Read the model definition and answer for the solid it produces. Units are mm, in the model's axes. Coordinates: 2 decimals unless noted, no trailing zeros. Write each loop counter-clockwise with the first axis right and the second up, starting at its lowest first coordinate (ties: lowest second). Pieces come first, ordered by that corner, then holes. Notation, with made-up numbers: (62.25, 30.25) -> (96.25, 30.25) arc R30 ccw to (96.25, 60.25) -> close; hole circle Ø1 at (42, 54). An arc over 180 degrees is marked (long way). Use CSV: the item, a comma, the result in double quotes.
from build123d import *

# Parameters (mm, degrees)
F0_W     = 13
F0_H     = 13
F1_DEPTH = 30
F2_SIZE  = 12.99999
F3_R     = 6.49999
F4_R     = 3
F5_DEPTH = 25
F6_SIZE  = 0.4


# Not quite as in the source:
# - a fillet or chamfer is up to 0.001 mm smaller than in the source, because OpenCascade refuses the exact size


with BuildPart() as f1:
    # F0 (on Top) → F1 (new body)
    with BuildSketch(Plane.XY):
        Rectangle(F0_W, F0_H)
    extrude(amount=F1_DEPTH)

    # F2 (size 13 in the source; OpenCascade refuses exactly that, so slightly less here)
    f2_edges = [f1.edges().sort_by_distance(p)[0] for p in [
        (0, -6.5, 0),
    ]]
    chamfer(f2_edges, length=F2_SIZE)

    # F3 (radius 6.5 in the source; OpenCascade refuses exactly that, so slightly less here)
    f3_edges = [f1.edges().sort_by_distance(p)[0] for p in [
        (6.5, 0, 30),
        (-6.5, 0, 30),
    ]]
    fillet(f3_edges, radius=F3_R)

    # F4 (on face) → F5 (cut)
    with BuildSketch(Plane(origin=(0, 6.5, 0), x_dir=(-1, 0, 0), z_dir=(0, 1, 0))):
        with Locations((0, 23.5)):
            Circle(F4_R)
    extrude(amount=-F5_DEPTH, mode=Mode.SUBTRACT)

    # F6
    f6_edges = [f1.edges().sort_by_distance(p)[0] for p in [
        (4.596197, 6.5, 28.096197),
        (4.596197, -6.5, 28.096197),
        (3, 6.5, 23.5),
        (3, -6.5, 23.5),
    ]]
    chamfer(f6_edges, length=F6_SIZE)


solid = f1.part
1. This flat-tipped pin is pushed along its axis until it touches: pin 1 Ø1.5 at (x, z) = (1, 9) entering from -Y. Where does it stop, or does it pass through?
Solutions:
pin 1,"stops at y = -3.25"
2. A cutting plane is placed at C-C (z = 2). Give the vertices of the cut face in (x, y), and give its area (3 significant figures).
Solutions:
outline,"(-6.5, 4.5) -> (6.5, 4.5) -> (6.5, 6.1) -> (6.1, 6.5) -> (-6.1, 6.5) -> (-6.5, 6.1) -> close"
area,"25.8 mm^2"
3. Find the intervals of material crossed by line 1 along Z through (x, y) = (0, 3.5); line 2 along Z through (x, y) = (-2.25, -4); line 3 along Y through (x, z) = (1.5, 6.5), in increasing order.
Solutions:
line 1,"z = 3 to 20.5, 26.5 to 30"
line 2,"z = 10.5 to 21.52, 25.48 to 29.6"
line 3,"y = 0 to 6.5"
4. A cutting plane is placed at D-D (z = 9). Give the vertices of the cut face in (x, y), and give its area (3 significant figures).
Solutions:
outline,"(-6.5, -2.5) -> (6.5, -2.5) -> (6.5, 6.1) -> (6.1, 6.5) -> (-6.1, 6.5) -> (-6.5, 6.1) -> close"
area,"117 mm^2"
5. For a pull along Z with two mould halves and no side action, classify faces 1 (the conical face through (-4.442, 6.386, 27.845)), 2 (the cylindrical face through (0.65, 0.09, 20.57)), 3 (the flat face through (0, -6.5, 19)) as pulls with the +Z half, pulls with the -Z half, needs draft (parallel to the pull), parting line crosses it, or undercut.
Solutions:
face 1,"pulls with the +Z half"
face 2,"undercut"
face 3,"needs draft"
